Geometry: final body of the model. Coordinates: model frame, mm. Coordinates: 2 decimals unless noted, no trailing zeros. Write each loop counter-clockwise with the first axis right and the second up, starting at its lowest first coordinate (ties: lowest second). Pieces come first, ordered by that corner, then holes.
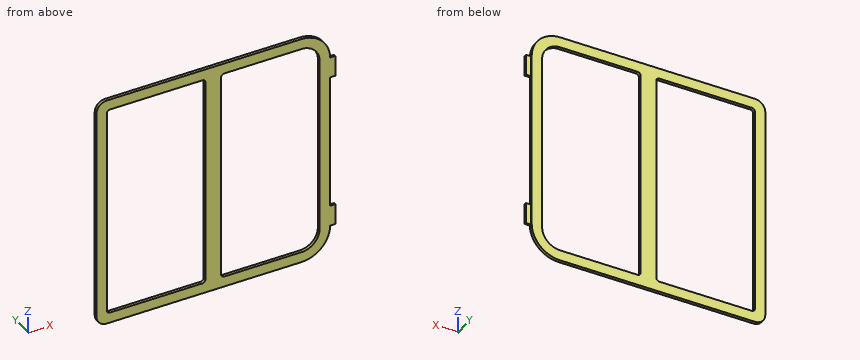
from build123d import *

# Parameters (mm, degrees)
F0_W     = 10
F0_H     = 40
F0_W_2   = 6
F0_W_3   = 14
F0_H_2   = 258
F1_DEPTH = 6
F2_DEPTH = 2


with BuildPart() as f1:
    # F0 (on Front) → F1 (new body)
    with BuildSketch(Plane.XZ):
        with BuildLine():
            Line((185.575712414, 225.5297148285), (-187.424287586, 225.5297148285))
            ThreePointArc((-187.424287586, 225.5297148285), (-201.5664232098, 219.6718504522), (-207.424287586, 205.5297148285))
            Line((-207.424287586, 205.5297148285), (-207.424287586, -202.4702851715))
            ThreePointArc((-207.424287586, -202.4702851715), (-201.5664232098, -216.6124207953), (-187.424287586, -222.4702851715))
            Line((-187.424287586, -222.4702851715), (185.575712414, -222.4702851715))
            ThreePointArc((185.575712414, -222.4702851715), (224.4665853792, -206.3611581368), (240.575712414, -167.4702851715))
            Line((240.575712414, -167.4702851715), (234.575712414, -167.4702851715))
            ThreePointArc((234.575712414, -167.4702851715), (220.2239446921, -202.1185174497), (185.575712414, -216.4702851715))
            Line((185.575712414, -216.4702851715), (-187.424287586, -216.4702851715))
            ThreePointArc((-187.424287586, -216.4702851715), (-197.3237825226, -212.3697801081), (-201.424287586, -202.4702851715))
            Line((-201.424287586, -202.4702851715), (-201.424287586, 205.5297148285))
            ThreePointArc((-201.424287586, 205.5297148285), (-197.3237825226, 215.4292097651), (-187.424287586, 219.5297148285))
            Line((-187.424287586, 219.5297148285), (185.575712414, 219.5297148285))
            ThreePointArc((185.575712414, 219.5297148285), (220.2239446921, 205.1779471066), (234.575712414, 170.5297148285))
            Line((234.575712414, 170.5297148285), (240.575712414, 170.5297148285))
            ThreePointArc((240.575712414, 170.5297148285), (224.4665853792, 209.4205877937), (185.575712414, 225.5297148285))
        make_face()
        with BuildLine():
            Line((220.575712414, 170.5297148285), (234.575712414, 170.5297148285))
            ThreePointArc((234.575712414, 170.5297148285), (220.2239446921, 205.1779471066), (185.575712414, 219.5297148285))
            Line((185.575712414, 219.5297148285), (-187.424287586, 219.5297148285))
            ThreePointArc((-187.424287586, 219.5297148285), (-197.3237825226, 215.4292097651), (-201.424287586, 205.5297148285))
            Line((-201.424287586, 205.5297148285), (-201.424287586, -202.4702851715))
            ThreePointArc((-201.424287586, -202.4702851715), (-197.3237825226, -212.3697801081), (-187.424287586, -216.4702851715))
            Line((-187.424287586, -216.4702851715), (185.575712414, -216.4702851715))
            ThreePointArc((185.575712414, -216.4702851715), (220.2239446921, -202.1185174497), (234.575712414, -167.4702851715))
            Line((234.575712414, -167.4702851715), (220.575712414, -167.4702851715))
            ThreePointArc((220.575712414, -167.4702851715), (211.315135886, -191.295361085), (188.325712414, -202.4702851715))
            Line((188.325712414, -202.4702851715), (37.575712414, -202.4702851715))
            ThreePointArc((37.575712414, -202.4702851715), (33.3330717268, -200.7129258587), (31.575712414, -196.4702851715))
            Line((31.575712414, -196.4702851715), (31.575712414, 199.5297148285))
            ThreePointArc((31.575712414, 199.5297148285), (33.3330717268, 203.7723555156), (37.575712414, 205.5297148285))
            Line((37.575712414, 205.5297148285), (188.325712414, 205.5297148285))
            ThreePointArc((188.325712414, 205.5297148285), (211.315135886, 194.354790742), (220.575712414, 170.5297148285))
        make_face()
        with BuildLine():
            Line((-187.424287586, -196.4702851715), (-187.424287586, 199.5297148285))
            ThreePointArc((-187.424287586, 199.5297148285), (-185.6669282732, 203.7723555156), (-181.424287586, 205.5297148285))
            Line((-181.424287586, 205.5297148285), (-4.424287586, 205.5297148285))
            ThreePointArc((-4.424287586, 205.5297148285), (-0.1816468989, 203.7723555156), (1.575712414, 199.5297148285))
            Line((1.575712414, 199.5297148285), (1.575712414, -196.4702851715))
            ThreePointArc((1.575712414, -196.4702851715), (-0.1816468989, -200.7129258587), (-4.424287586, -202.4702851715))
            Line((-4.424287586, -202.4702851715), (-181.424287586, -202.4702851715))
            ThreePointArc((-181.424287586, -202.4702851715), (-185.6669282732, -200.7129258587), (-187.424287586, -196.4702851715))
        make_face(mode=Mode.SUBTRACT)
        with Locations((245.575712414, 150.5297148285)):
            Rectangle(F0_W, F0_H)
        with Locations((237.575712414, 150.5297148285)):
            Rectangle(F0_W_2, F0_H)
        with Locations((227.575712414, 150.5297148285)):
            Rectangle(F0_W_3, F0_H)
        with Locations((227.575712414, 1.5297148285)):
            Rectangle(F0_W_3, F0_H_2)
        with Locations((237.575712414, 1.5297148285)):
            Rectangle(F0_W_2, F0_H_2)
        with Locations((237.575712414, -147.4702851715)):
            Rectangle(F0_W_2, F0_H)
        with Locations((227.575712414, -147.4702851715)):
            Rectangle(F0_W_3, F0_H)
        with Locations((245.575712414, -147.4702851715)):
            Rectangle(F0_W, F0_H)
    extrude(amount=F1_DEPTH)

    # F0 (on Front) → F2 (cut)
    with BuildSketch(Plane.XZ):
        with Locations((245.575712414, 150.5297148285)):
            Rectangle(F0_W, F0_H)
        with Locations((245.575712414, -147.4702851715)):
            Rectangle(F0_W, F0_H)
    extrude(amount=F2_DEPTH, mode=Mode.SUBTRACT)


solid = f1.part
Item 1: Section A-A, the plane z = 74. Output: boundary loops of the cut face in (x, y), plus the area to 3 significant figures.
Derived:
outline: (-207.42, -6) - (-187.42, -6) - (-187.42, 0) - (-207.42, 0) - close; (1.58, -6) - (31.58, -6) - (31.58, 0) - (1.58, 0) - close; (220.58, -6) - (240.58, -6) - (240.58, 0) - (220.58, 0) - close
area: 420 mm2
Item 2: Section B-B, the plane x = 95. Output: boundary loops of the cut face in (y, z).
Derived:
outline: (-6, -222.47) - (0, -222.47) - (0, -202.47) - (-6, -202.47) - close; (-6, 205.53) - (0, 205.53) - (0, 225.53) - (-6, 225.53) - close
Item 3: Pin query (flat end, axial travel): pin 1 (2 mm diameter, centred on y = -5, z = -79, fed in from +X); pin 2 (1.2 mm diameter, centred on x = 244.5, y = -3, fed in from +Z); pin 3 (8 mm diameter, centred on x = 247.5, z = 158.5, fed in from +Y). Return the tip coordinate at first contact, or that it passes through.
Derived:
pin 1: stops at x = 240.58
pin 2: stops at z = 170.53
pin 3: stops at y = -2
Item 4: Material intervals for probe 1 along X at (y, z) = (-2.8, 65); probe 2 along X at (y, z) = (-3.15, -162); probe 3 along Z at (x, y) = (70, -5.05), sorted ascending.
Derived:
probe 1: x = -207.42 to -187.42, 1.58 to 31.58, 220.58 to 240.58
probe 2: x = -207.42 to -187.42, 1.58 to 31.58, 220.58 to 250.58
probe 3: z = -222.47 to -202.47, 205.53 to 225.53
Item 5: Section C-C, the plane y = -3.25. State how many separate pieces and enclosed holes the cut face has, plus the area to 3 significant figures.
Derived:
separate pieces: 1
enclosed holes: 2
area: 46,400 mm2
Item 6: Section D-D, the plane z = -151. Output: boundary loops of the cut face in (x, y), plus the area to 3 significant figures.
Derived:
outline: (-207.42, -6) - (-187.42, -6) - (-187.42, 0) - (-207.42, 0) - close; (1.58, -6) - (31.58, -6) - (31.58, 0) - (1.58, 0) - close; (220.58, -6) - (250.58, -6) - (250.58, -2) - (240.58, -2) - (240.58, 0) - (220.58, 0) - close
area: 460 mm2
